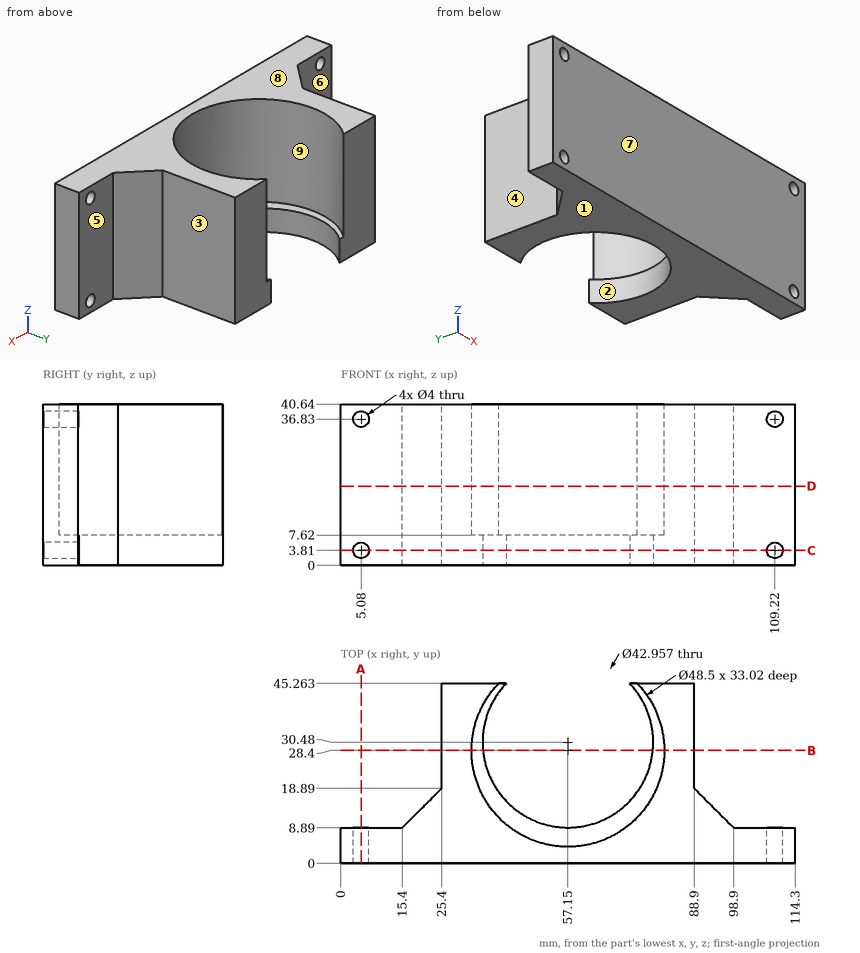
Could you check a few things on this drawing? It's one solid part, dimensions in mm from its lowest x, y, z. A direction names the side the tool comes from. Round coordinates to 2 decimals unless told otherwise and drop trailing zeros. Order: outer loops, then holes, each group sorted by start corner. A loop starts at its lowest first (then second) coordinate and runs counter-clockwise, first axis right, second up. Notation, with made-up numbers: M 74,-6.5 L 87,-6.5 A30 cw 87,16.5 Z; hole C -39,12.25 d9. An arc over 180 degrees is marked long. Return JSON: item names as keys, results as strings. Group by question number.
1. If we mould it in two halves opening along X, with no side actions, what happens to the marked faces 1, 2, 3 and 4? For each: pulls with the +X half, pulls with the -X half, needs draft (parallel to the pull), parting line crosses it, or undercut.
2. I'm going to push flat-ended pins straight in: pin 1 Ø1.5 at (x, z) = (17.5, 4.5) entering from +Y; pin 2 Ø3.5 at (x, z) = (5.08, 36.83) entering from +Y; pin 3 Ø3 at (x, z) = (100, 30) entering from +Y; pin 4 Ø5 at (x, z) = (5.08, 3.81) entering from +Y. Where does each tip first touch, or does it pass through?
3. Please list where these lines run through material, in increasing order: probe 1 along X at (y, z) = (2.5, 36.83); probe 2 along Z at (x, y) = (5, 5); probe 3 along X at (y, z) = (30, 2).
4. If we section it at A-A on x = 5.08: List the corners of the cut face in (y, z) for me.
5. On a 3-axis mill with a long thin cutter (end or side, diameter ignored), from which of +Z, -Z, +X, -X, +Y, -Y can I reach the whole of each face in a straight line? I mean the marked faces 5, 6, 7, 8 and 9. Say none if no direction works.
6. If we section it at C-C on z = 3.81: List the corners of the cut face in (x, y) for me, then the cut area to 3 significant figures.
7. If we section it at B-B on y = 28.4: List the corners of the cut face in (x, z) for me.
8. If we section it at D-D on z = 20: List the corners of the cut face in (x, y) for me, then the cut area to 3 significant figures.
Reply:
{
 "1": {"face 1": "needs draft", "face 2": "undercut", "face 3": "pulls with the +X half", "face 4": "pulls with the -X half"},
 "2": {"pin 1": "y = 11.74", "pin 2": "through", "pin 3": "y = 9.29", "pin 4": "y = 8.89"},
 "3": {"probe 1": "0 to 3.08, 7.08 to 107.22, 111.22 to 114.3", "probe 2": "0 to 1.81, 5.81 to 34.83, 38.83 to 40.64", "probe 3": "25.4 to 35.68, 78.62 to 88.9"},
 "4": {"outline": "M 0,0 L 8.89,0 L 8.89,1.81 L 0,1.81 Z; M 0,5.81 L 8.89,5.81 L 8.89,34.83 L 0,34.83 Z; M 0,38.83 L 8.89,38.83 L 8.89,40.64 L 0,40.64 Z"},
 "5": {"face 5": "+Z, -Z, +X, +Y", "face 6": "+Z, -Z, -X, +Y", "face 7": "+Z, -Z, +X, -X, -Y", "face 8": "+Z, +X, -X, +Y, -Y", "face 9": "+Z"},
 "6": {"outline": "M 0,0 L 3.08,0 L 3.08,8.89 L 0,8.89 Z; M 7.08,0 L 107.22,0 L 107.22,8.89 L 98.9,8.89 L 88.9,18.89 L 88.9,45.26 L 72.73,45.26 A21.48 cw long 41.57,45.26 L 25.4,45.26 L 25.4,18.89 L 15.4,8.89 L 7.08,8.89 Z; M 111.22,0 L 114.3,0 L 114.3,8.89 L 111.22,8.89 Z", "area": "2,050 mm^2"},
 "7": {"outline": "M 25.4,0 L 35.77,0 L 35.77,7.62 L 32.9,7.62 L 32.9,40.64 L 25.4,40.64 Z; M 78.53,0 L 88.9,0 L 88.9,40.64 L 81.4,40.64 L 81.4,7.62 L 78.53,7.62 Z"},
 "8": {"outline": "M 0,0 L 114.3,0 L 114.3,8.89 L 98.9,8.89 L 88.9,18.89 L 88.9,45.26 L 74.58,45.26 A24.25 cw long 39.72,45.26 L 25.4,45.26 L 25.4,18.89 L 15.4,8.89 L 0,8.89 Z", "area": "1,760 mm^2"}
}
